Check sheet for the modelled part. Datum: model origin and axes. Units: mm. Face numbers are marked on the shaded views. Round coordinates to 2 decimals unless told otherwise and drop trailing zeros. Order: outer loops, then holes, each group sorted by start corner. A loop starts at its lowest first (then second) coordinate and runs counter-clockwise, first axis right, second up. Notation, with made-up numbers: M -17.5,47.5 L 5.5,47.5 A11 cw 5.5,64.5 Z; hole C -39,7.5 d11. An arc over 180 degrees is marked long. One line per item, written item: value. Start each with the question number.
(1) Cross-section at D-D, the plane y = -66. Enter the section's corners in (x, z).
(2) Cross-section at C-C, the plane x = -48. Enter the section's corners in (y, z).
(3) Thickness scan on L1, parallel to Z at x = 0.8, y = -4; L2, parallel to X at y = -93, z = 7.25; L3, parallel to Y at x = -53.5, z = 6.75. Record the ranges inside material, lowest first.
(4) Cross-section at A-A, the plane y = -4. Enter the section's corners in (x, z), and give its area (3 significant figures).
(5) Cross-section at B-B, the plane z = 4. Enter the section's corners in (x, y), and give its area (3 significant figures).
(6) Release check for a two-part mould opening along Y. For the marked faces 1, 2 and 3 record: released by +Y, released by -Y, zero draft, split by the parting line, or undercut.
(7) Depth check by flat-ended pin: pin 1 Ø2 at (y, z) = (-44, 7) entering from +X; pin 2 Ø0.8 at (y, z) = (-99, 6) entering from +X; pin 3 Ø2.5 at (y, z) = (-96, 2) entering from +X. Enter the tip coordinate at first touch or a pass-through.
from build123d import *

# Parameters (mm, degrees)
BOSS_EXTRUDE1_DEPTH = 8
SKETCH2_R           = 2
CUT_EXTRUDE1_DEPTH  = 117.079972433


with BuildPart() as part:
    # Sketch1 → Boss-Extrude1 (new body)
    with BuildSketch(Plane.XY):
        Polygon((0, 0), (0, -8), (-58.4, -89.485853422), (-58.4, -100), (-52.4, -100), (-52.4, -98.4), (-56.8, -98.4), (-56.8, -90), (1.6, -8.514146578), (1.6, 0), align=None)
    extrude(amount=BOSS_EXTRUDE1_DEPTH)

    # Sketch2 → Cut-Extrude1 (cut, through all)
    with BuildSketch(Plane.ZY):
        with Locations(Location((4, -4, 0), (0, 0, 270))):
            Circle(SKETCH2_R)
        Polygon((0, 0), (0, -2.343145751), (2.343145751, 0), align=None)
        Polygon((8, -2.343145751), (5.656854249, 0), (8, 0), align=None)
    extrude(amount=-CUT_EXTRUDE1_DEPTH, mode=Mode.SUBTRACT)


solid = part.part
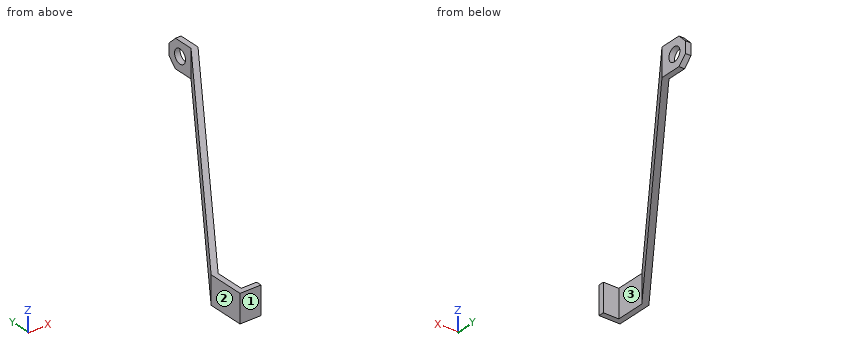
Values found:
1. outline: M -41.57,0 L -39.6,0 L -39.6,8 L -41.57,8 Z
2. outline: M -77.72,0 L -74.97,0 L -74.97,8 L -77.72,8 Z
3. L1: 0 to 2, 6 to 8
3. L2: -58.4 to -56.8
3. L3: -100 to -98.4, -85.4 to -82.65
4. outline: M 0,0 L 1.6,0 L 1.6,2 L 0,2 Z; M 0,6 L 1.6,6 L 1.6,8 L 0,8 Z
4. area: 6.40 mm^2
5. outline: M -58.4,-100 L -52.4,-100 L -52.4,-98.4 L -56.8,-98.4 L -56.8,-90 L 1.6,-8.51 L 1.6,-6 L 0,-6 L 0,-8 L -58.4,-89.49 Z; M 0,-2 L 1.6,-2 L 1.6,0 L 0,0 Z
5. area: 191 mm^2
6. face 1: released by -Y
6. face 2: zero draft
6. face 3: undercut
7. pin 1: x = -23.12
7. pin 2: x = -52.4
7. pin 3: x = -56.8
